from build123d import *

# Parameters (mm, degrees)
SKETCH1_W                      = 1.5875
SKETCH1_H                      = 152.4
BASE_FLANGE1_DEPTH             = 355.6
EDGE_FLANGE1_STRIP_W           = 7.8232
EDGE_FLANGE1_STRIP_H           = 1.5875
EDGE_FLANGE1_STRIP_CUT_DEPTH   = 355.6
EDGE_FLANGE1_STRIP_2_W         = 7.8232
EDGE_FLANGE1_STRIP_2_H         = 1.5875
EDGE_FLANGE1_STRIP_CUT_2_DEPTH = 355.6
EDGE_FLANGE1_DEPTH             = 355.6
EDGE_FLANGE1_BEND_DEPTH        = 355.6
EDGE_FLANGE2_STRIP_W           = 7.8232
EDGE_FLANGE2_STRIP_H           = 1.5875
EDGE_FLANGE2_STRIP_CUT_DEPTH   = 355.6
EDGE_FLANGE2_STRIP_2_W         = 7.8232
EDGE_FLANGE2_STRIP_2_H         = 1.5875
EDGE_FLANGE2_STRIP_CUT_2_DEPTH = 355.6
EDGE_FLANGE2_DEPTH             = 355.6
EDGE_FLANGE2_BEND_DEPTH        = 355.6


# Sheet-metal steps are written as plain solids
with BuildPart() as part:
    # Sketch1 → Base-Flange1 (new body)
    with BuildSketch(Plane(origin=(0, 0, 0), x_dir=(0, 0, -1), z_dir=(1, 0, 0))):
        with Locations((0.79375, 76.2)):
            Rectangle(SKETCH1_W, SKETCH1_H)
    extrude(amount=BASE_FLANGE1_DEPTH)

    # Edge-Flange1 strip (across the edge) → Edge-Flange1 strip cut (cut)
    with BuildSketch(Plane(origin=(355.6, 152.4, 0), x_dir=(0, -1, 0), z_dir=(-1, 0, 0))):
        with Locations((-3.175, -0.79375)):
            Rectangle(EDGE_FLANGE1_STRIP_W, EDGE_FLANGE1_STRIP_H)
    extrude(amount=EDGE_FLANGE1_STRIP_CUT_DEPTH, mode=Mode.SUBTRACT)

    # Edge-Flange1 strip 2 (across the edge) → Edge-Flange1 strip cut 2 (cut)
    with BuildSketch(Plane.YZ):
        with Locations((-3.175, -0.79375)):
            Rectangle(EDGE_FLANGE1_STRIP_2_W, EDGE_FLANGE1_STRIP_2_H)
    extrude(amount=EDGE_FLANGE1_STRIP_CUT_2_DEPTH, mode=Mode.SUBTRACT)

    # Edge-Flange1 section (across the edge) → Edge-Flange1 (add)
    with BuildSketch(Plane(origin=(355.6, 152.4, 0), x_dir=(0, -1, 0), z_dir=(-1, 0, 0))):
        with BuildLine():
            Line((-1.5875, 0.7366), (-1.5875, 112.7125))
            Line((-1.5875, 112.7125), (0, 112.7125))
            Line((0, 112.7125), (0, 0.7366))
            ThreePointArc((0, 0.7366), (0.215745145, 0.215745145), (0.7366, 0))
            Line((0.7366, 0), (0.7366, -1.5875))
            ThreePointArc((0.7366, -1.5875), (-0.90678687, -0.90678687), (-1.5875, 0.7366))
        make_face()
    extrude(amount=EDGE_FLANGE1_DEPTH)

    # Edge-Flange1 section 2 (across the edge) → Edge-Flange1 bend (add)
    with BuildSketch(Plane.YZ):
        with BuildLine():
            Line((-1.5875, 0.7366), (-1.5875, 112.7125))
            Line((-1.5875, 112.7125), (0, 112.7125))
            Line((0, 112.7125), (0, 0.7366))
            ThreePointArc((0, 0.7366), (0.215745145, 0.215745145), (0.7366, 0))
            Line((0.7366, 0), (0.7366, -1.5875))
            ThreePointArc((0.7366, -1.5875), (-0.90678687, -0.90678687), (-1.5875, 0.7366))
        make_face()
    extrude(amount=EDGE_FLANGE1_BEND_DEPTH)

    # Edge-Flange2 strip (across the edge) → Edge-Flange2 strip cut (cut)
    with BuildSketch(Plane(origin=(0, 153.9875, 112.7125), x_dir=(0, 0, -1), z_dir=(1, 0, 0))):
        with Locations((-3.175, -0.79375)):
            Rectangle(EDGE_FLANGE2_STRIP_W, EDGE_FLANGE2_STRIP_H)
    extrude(amount=EDGE_FLANGE2_STRIP_CUT_DEPTH, mode=Mode.SUBTRACT)

    # Edge-Flange2 strip 2 (across the edge) → Edge-Flange2 strip cut 2 (cut)
    with BuildSketch(Plane(origin=(355.6, -1.5875, 112.7125), x_dir=(0, 0, -1), z_dir=(-1, 0, 0))):
        with Locations((-3.175, -0.79375)):
            Rectangle(EDGE_FLANGE2_STRIP_2_W, EDGE_FLANGE2_STRIP_2_H)
    extrude(amount=EDGE_FLANGE2_STRIP_CUT_2_DEPTH, mode=Mode.SUBTRACT)

    # Edge-Flange2 section (across the edge) → Edge-Flange2 (add)
    with BuildSketch(Plane(origin=(0, 153.9875, 112.7125), x_dir=(0, 0, -1), z_dir=(1, 0, 0))):
        with BuildLine():
            Line((-1.5875, 0.7366), (-1.5875, 23.8125))
            Line((-1.5875, 23.8125), (0, 23.8125))
            Line((0, 23.8125), (0, 0.7366))
            ThreePointArc((0, 0.7366), (0.215745145, 0.215745145), (0.7366, 0))
            Line((0.7366, 0), (0.7366, -1.5875))
            ThreePointArc((0.7366, -1.5875), (-0.90678687, -0.90678687), (-1.5875, 0.7366))
        make_face()
    extrude(amount=EDGE_FLANGE2_DEPTH)

    # Edge-Flange2 section 2 (across the edge) → Edge-Flange2 bend (add)
    with BuildSketch(Plane(origin=(355.6, -1.5875, 112.7125), x_dir=(0, 0, -1), z_dir=(-1, 0, 0))):
        with BuildLine():
            Line((-1.5875, 0.7366), (-1.5875, 23.8125))
            Line((-1.5875, 23.8125), (0, 23.8125))
            Line((0, 23.8125), (0, 0.7366))
            ThreePointArc((0, 0.7366), (0.215745145, 0.215745145), (0.7366, 0))
            Line((0.7366, 0), (0.7366, -1.5875))
            ThreePointArc((0.7366, -1.5875), (-0.90678687, -0.90678687), (-1.5875, 0.7366))
        make_face()
    extrude(amount=EDGE_FLANGE2_BEND_DEPTH)


solid = part.part
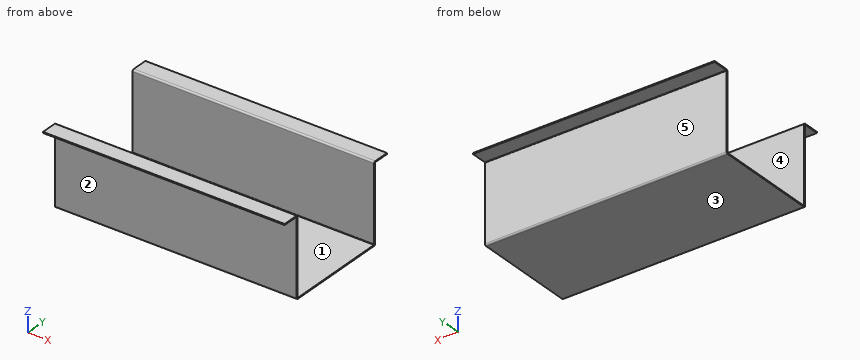
Here's how the part is built. I have some questions about the finished solid (model axes, mm). Face numbers are marked on the shaded views. A direction names the side the tool comes from. Coordinates: 2 decimals unless noted, no trailing zeros. Write each loop counter-clockwise with the first axis right and the second up, starting at its lowest first coordinate (ties: lowest second). Pieces come first, ordered by that corner, then holes. Notation, with made-up numbers: (70, 11) - (83, 11) arc R16 cw to (83, 27) - close; hole circle Ø10 at (24, 82). An arc over 180 degrees is marked (long way). Use one line per item in the form item = value.
1) Suppose I cut it at A-A, the plane z = 51.5. Write out the boundary of the cut face in (x, y).
Solved:
outline = (0, -1.59) - (355.6, -1.59) - (355.6, 0) - (0, 0) - close; (0, 152.4) - (355.6, 152.4) - (355.6, 153.99) - (0, 153.99) - close
2) I'm going to push flat-ended pins straight in: P1, Ø4, axis at x = 66.5, z = 63, coming from the -Y side; P2, Ø18.5, axis at x = 124, y = -19, coming from the -Z side. Where does each tip first touch, or does it pass through?
Solved:
P1 = -1.59
P2 = 112.71
3) I need wall thicknesses on line 1 (Y direction, x = 69, z = 87); line 2 (Z direction, x = 98.5, y = 140.5); line 3 (Z direction, x = 196, y = 152). Which ranges of each line are inside material? Lowest first, please.
Solved:
line_1 = -1.59 to 0, 152.4 to 153.99
line_2 = -1.59 to 0
line_3 = -1.56 to 0.08
4) Thinking about a two-plate mould opening in Y: for the marked faces 1, 2 and 3, which applies, released by +Y, released by -Y, zero draft, split by the parting line, or undercut?
Solved:
face_1 = undercut
face_2 = released by -Y
face_3 = zero draft
5) Suppose I cut it at C-C, the plane y = -9.5. Write out the boundary of the cut face in (x, z).
Solved:
outline = (0, 112.71) - (355.6, 112.71) - (355.6, 114.3) - (0, 114.3) - close
6) Suppose I cut it at B-B, the plane x = 88. Write out the boundary of the cut face in (y, z), plus the area to 3 significant figures.
Solved:
outline = (-25.4, 112.71) - (-2.32, 112.71) arc R0.74 cw to (-1.59, 111.98) - (-1.59, 0.74) arc R2.32 ccw to (0.74, -1.59) - (151.66, -1.59) arc R2.32 ccw to (153.99, 0.74) - (153.99, 111.98) arc R0.74 cw to (154.72, 112.71) - (177.8, 112.71) - (177.8, 114.3) - (154.72, 114.3) arc R2.32 ccw to (152.4, 111.98) - (152.4, 0.74) arc R0.74 cw to (151.66, 0) - (0.74, 0) arc R0.74 cw to (0, 0.74) - (0, 111.98) arc R2.32 ccw to (-2.32, 114.3) - (-25.4, 114.3) - close
area = 681 mm2
7) On a 3-axis mill with a long thin cutter (end or side, diameter ignored), from which of +Z, -Z, +X, -X, +Y, -Y can I reach the whole of each face in a straight line? I mean the marked faces 4 and 5. Say none if no direction works.
Solved:
face_4 = +Z, +X, -X
face_5 = -Z, +X, -X, +Y
